Here's how the part is built. I have some questions about the finished solid (model axes, mm). A direction names the side the tool comes from. Give positions to 0.01 mm unless a question says otherwise; leave off trailing zeros. Loops run counter-clockwise (first coordinate to the right, second up) from the corner with the lowest first, then second, coordinate; pieces in that order, holes last. Notation, with made-up numbers: (-10, -4) - (9, -4) arc R25 cw to (9, 25) - close; hole circle Ø2 at (58.25, -26.5). An arc over 180 degrees is marked (long way). Use a Markdown table: item, result.
from build123d import *

# Parameters (mm, degrees)
SKETCH1_W                        = 113
SKETCH1_H                        = 107
MAIN_BODY_DEPTH                  = 5
SKETCH19_W                       = 18.5
SKETCH19_H                       = 18.5
BOSS_EXTRUDE1_DEPTH              = 3
SKETCH7_R                        = 3.5
SKETCH7_W                        = 80
SKETCH7_H                        = 51.5
SCREEN_AND_KNOB_LOCATATION_DEPTH = 79.220841213
SKETCH11_W                       = 67.654258951
SKETCH11_H                       = 30.527744354
INTERNAL_CAVITY_DEPTH            = 3
BOARDERS_OUTLINE_W               = 113
BOARDERS_OUTLINE_H               = 107
BOARDERS_DEPTH                   = 15
SKETCH6_R                        = 3.5
SCREW_HEAD_PLACEMENT_DEPTH       = 15
SKETCH10_R                       = 1.68009103
SKETCH10_R_2                     = 2
SCREW_HOLE_THROUGH_DEPTH         = 80.243296246
SKETCH14_W                       = 4.25
SKETCH14_H                       = 28
SD_CARD_SLOT_DEPTH               = 10
SKETCH15_R                       = 3
BUTTON_PRESS_DEPTH               = 8.25
GROOVE_CUT_DEPTH                 = 80.865511956
CANCEL_DECAL_DEPTH               = 1
MAIN_BODY_FILLET_R               = 4
SKETCH18_R                       = 7.625
CUT_EXTRUDE1_DEPTH               = 6.5


# Read off the part's stored shape, not the designer's step: Boarders
with BuildPart() as part:
    # Sketch1 → Main Body (new body)
    with BuildSketch(Plane.XY):
        Rectangle(SKETCH1_W, SKETCH1_H)
    extrude(amount=MAIN_BODY_DEPTH)

    # Sketch19 → Boss-Extrude1 (add)
    with BuildSketch(Plane(origin=(0, 0, 0), x_dir=(-1, 0, 0), z_dir=(0, 0, -1))):
        with Locations((-36.5, -34.5)):
            Rectangle(SKETCH19_W, SKETCH19_H)
    extrude(amount=BOSS_EXTRUDE1_DEPTH)

    # Sketch7 → Screen and knob locatation (cut, through all)
    with BuildSketch(Plane.XY.offset(5)):
        with Locations((36.3, -34.31)):
            Circle(SKETCH7_R)
        with Locations((-0.5, 9.25)):
            Rectangle(SKETCH7_W, SKETCH7_H)
    extrude(amount=-SCREEN_AND_KNOB_LOCATATION_DEPTH, mode=Mode.SUBTRACT)

    # Sketch11 → Internal cavity (cut)
    with BuildSketch(Plane(origin=(0, 0, 0), x_dir=(-1, 0, 0), z_dir=(0, 0, -1))):
        with Locations((6.575112586, -34.017474747)):
            Rectangle(SKETCH11_W, SKETCH11_H)
    extrude(amount=-INTERNAL_CAVITY_DEPTH, mode=Mode.SUBTRACT)

    # Boarders outline → Boarders (add)
    with BuildSketch(Plane(origin=(0, 0, 0), x_dir=(-1, 0, 0), z_dir=(0, 0, -1))):
        Rectangle(BOARDERS_OUTLINE_W, BOARDERS_OUTLINE_H)
        Polygon((-27.25201689, -49.281346924), (-27.25201689, -44.5), (-47.5, -44.5), (-47.5, 44.5), (47.5, 44.5), (47.5, -44.5), (40.402242061, -44.5), (40.402242061, -49.281346924), align=None, mode=Mode.SUBTRACT)
    extrude(amount=BOARDERS_DEPTH)

    # Sketch6 → Screw Head Placement (cut)
    with BuildSketch(Plane.XY.offset(5)):
        with Locations((-51.5, 48.5)):
            Circle(SKETCH6_R)
        with Locations((-51.5, -48.5)):
            Circle(SKETCH6_R)
        with Locations((51.5, -48.5)):
            Circle(SKETCH6_R)
        with Locations((51.5, 48.5)):
            Circle(SKETCH6_R)
    extrude(amount=-SCREW_HEAD_PLACEMENT_DEPTH, mode=Mode.SUBTRACT)

    # Sketch10 → Screw hole through (cut, through all)
    with BuildSketch(Plane.XY.offset(-10)):
        with Locations((-51.5, 48.5)):
            Circle(SKETCH10_R)
        with Locations((51.5, 48.5)):
            Circle(SKETCH10_R)
        with Locations((51.5, -48.5)):
            Circle(SKETCH10_R)
        with Locations((-51.5, -48.5)):
            Circle(SKETCH10_R_2)
    extrude(amount=-SCREW_HOLE_THROUGH_DEPTH, mode=Mode.SUBTRACT)

    # Sketch14 → SD Card Slot (cut)
    with BuildSketch(Plane.ZY.offset(56.5)):
        with Locations((-12.875, 8)):
            Rectangle(SKETCH14_W, SKETCH14_H)
    extrude(amount=-SD_CARD_SLOT_DEPTH, mode=Mode.SUBTRACT)

    # Sketch15 → Button Press (add)
    with BuildSketch(Plane(origin=(0, 0, 3), x_dir=(-1, 0, 0), z_dir=(0, 0, -1))):
        with Locations((-3.7199, -35.4101)):
            Circle(SKETCH15_R)
    extrude(amount=BUTTON_PRESS_DEPTH)

    # Sketch16 → Groove Cut (cut, through all)
    with BuildSketch(Plane(origin=(0, 0, 3), x_dir=(-1, 0, 0), z_dir=(0, 0, -1))):
        with BuildLine():
            Line((2.2801, -39.4101), (7.826420717, -39.4101))
            Line((7.826420717, -39.4101), (7.826420717, -39.9101))
            Line((7.826420717, -39.9101), (2.729589743, -39.9101))
            ThreePointArc((2.729589743, -39.9101), (1.86123883, -41.346591673), (0.2801, -41.9101))
            Line((0.2801, -41.9101), (-7.7199, -41.9101))
            ThreePointArc((-7.7199, -41.9101), (-9.487666953, -41.177866953), (-10.2199, -39.4101))
            Line((-10.2199, -39.4101), (-10.2199, -31.4101))
            ThreePointArc((-10.2199, -31.4101), (-9.487666953, -29.642333047), (-7.7199, -28.9101))
            Line((-7.7199, -28.9101), (0.2801, -28.9101))
            ThreePointArc((0.2801, -28.9101), (1.86123883, -29.473608327), (2.729589743, -30.9101))
            Line((2.729589743, -30.9101), (7.826420717, -30.9101))
            Line((7.826420717, -30.9101), (7.826420717, -31.4101))
            Line((7.826420717, -31.4101), (2.2801, -31.4101))
            ThreePointArc((2.2801, -31.4101), (1.694313562, -29.995886438), (0.2801, -29.4101))
            Line((0.2801, -29.4101), (-7.7199, -29.4101))
            ThreePointArc((-7.7199, -29.4101), (-9.134113562, -29.995886438), (-9.7199, -31.4101))
            Line((-9.7199, -31.4101), (-9.7199, -39.4101))
            ThreePointArc((-9.7199, -39.4101), (-9.134113562, -40.824313562), (-7.7199, -41.4101))
            Line((-7.7199, -41.4101), (0.2801, -41.4101))
            ThreePointArc((0.2801, -41.4101), (1.694313562, -40.824313562), (2.2801, -39.4101))
        make_face()
    extrude(amount=-GROOVE_CUT_DEPTH, mode=Mode.SUBTRACT)

    # Sketch17 → CAncel Decal (cut)
    with BuildSketch(Plane.XY.offset(5)):
        Polygon((0.356446609, -32.753753391), (3.012793219, -35.4101), (0.356446609, -38.066446609), (1.063553391, -38.773553391), (3.7199, -36.117206781), (6.376246609, -38.773553391), (7.083353391, -38.066446609), (4.427006781, -35.4101), (7.083353391, -32.753753391), (6.376246609, -32.046646609), (3.7199, -34.702993219), (1.063553391, -32.046646609), align=None)
    extrude(amount=-CANCEL_DECAL_DEPTH, mode=Mode.SUBTRACT)

    # Main Body Fillet
    main_body_fillet_edges = [part.edges().sort_by_distance(p)[0] for p in [
        (56.5, -53.5, -5),
        (-56.5, -53.5, -5),
        (-56.5, 53.5, -5),
        (56.5, 53.5, -5),
    ]]
    fillet(main_body_fillet_edges, radius=MAIN_BODY_FILLET_R)

    # Sketch18 → Cut-Extrude1 (cut)
    with BuildSketch(Plane.XY.offset(5)):
        with Locations((36.3, -34.31)):
            Circle(SKETCH18_R)
    extrude(amount=-CUT_EXTRUDE1_DEPTH, mode=Mode.SUBTRACT)


solid = part.part
(1) On a 3-axis mill with a long thin cutter (end or side, diameter ignored), from which of +Z, -Z, +X, -X, +Y, -Y can I reach the whole of each face in a straight line? I mean faces 1 (the face through (27.25, -35, -1)), 2 (the face through (-54.08, 50.865, -2.395)), 3 (the face through (-40.5, 9, 3)). Say none if no direction works.
A:
| item | result |
|---|---|
| face 1 | -Z |
| face 2 | +Z |
| face 3 | +Z, -Z |
(2) Suppose I cut it at D-D on x = 30. Write out the boundary of the cut face in (y, z), plus the area to 3 significant figures.
A:
| item | result |
|---|---|
| outline | (-53.5, -15) - (-44.5, -15) - (-44.5, 0) - (-43.75, 0) - (-43.75, -3) - (-25.25, -3) - (-25.25, 0) - (-16.5, 0) - (-16.5, 5) - (-30.01, 5) - (-30.01, -1.5) - (-38.61, -1.5) - (-38.61, 5) - (-53.5, 5) - close; (35, 0) - (44.5, 0) - (44.5, -15) - (53.5, -15) - (53.5, 5) - (35, 5) - close |
| area | 547 mm2 |
(3) Will these pins go through, and if not, where does the flat tip stop? pin 1 (3.5 mm diameter, centred on x = -51, y = 50, fed in from +Z); pin 2 (9 mm diameter, centred on x = 38.5, y = -30.5, fed in from -Z); pin 3 (7 mm diameter, centred on x = -52.5, y = 11.5, fed in from -Z); pin 4 (8 mm diameter, centred on x = 26.5, y = 29, fed in from +Z).
A:
| item | result |
|---|---|
| pin 1 | z = -10 |
| pin 2 | z = -3 |
| pin 3 | z = -10.75 |
| pin 4 | through |
(4) Suppose I cut it at A-A on y = -2.5. Write out the boundary of the cut face in (x, z), plus the area to 3 significant figures.
A:
| item | result |
|---|---|
| outline | (-56.5, -10.75) - (-47.5, -10.75) - (-47.5, 0) - (-40.5, 0) - (-40.5, 5) - (-56.5, 5) - close; (39.5, 0) - (47.5, 0) - (47.5, -15) - (56.5, -15) - (56.5, 5) - (39.5, 5) - close |
| area | 397 mm2 |
(5) We'd pull the mould along X, two halves only. Please class faces 4 (the face through (-55.297, 52.359, -4.86)), 5 (the face through (-52, -6, -13)), 6 (the face through (-6, -18.754, 1)): pulls with the +X half, pulls with the -X half, needs draft (parallel to the pull), parting line crosses it, or undercut.
A:
| item | result |
|---|---|
| face 4 | pulls with the -X half |
| face 5 | needs draft |
| face 6 | undercut |
(6) Suppose I cut it at B-B on x = -15.5. Write out the boundary of the cut face in (y, z).
A:
| item | result |
|---|---|
| outline | (-53.5, -15) - (-49.28, -15) - (-49.28, 3) - (-18.75, 3) - (-18.75, 0) - (-16.5, 0) - (-16.5, 5) - (-53.5, 5) - close; (35, 0) - (44.5, 0) - (44.5, -15) - (53.5, -15) - (53.5, 5) - (35, 5) - close |
(7) If I drill on line 1 (Y direction, x = -51.5, z = -4.25); line 2 (Y direction, x = -39, z = 2); line 3 (Y direction, x = -39, z = -10.25), over which ranges is the centre line in solid material (lowest first)?
A:
| item | result |
|---|---|
| line 1 | -53.5 to -52, -45 to 45, 52 to 53.5 |
| line 2 | -53.5 to -49.28, -18.75 to -16.5, 35 to 53.5 |
| line 3 | -53.5 to -49.28, 44.5 to 53.5 |
(8) Suppose I cut it at C-C on z = -12.5. Write out the boundary of the cut face in (x, y).
A:
| item | result |
|---|---|
| outline | (-56.5, -49.5) arc R4 ccw to (-52.5, -53.5) - (52.5, -53.5) arc R4 ccw to (56.5, -49.5) - (56.5, 49.5) arc R4 ccw to (52.5, 53.5) - (-52.5, 53.5) arc R4 ccw to (-56.5, 49.5) - (-56.5, 22) - (-47.5, 22) - (-47.5, 44.5) - (47.5, 44.5) - (47.5, -44.5) - (27.25, -44.5) - (27.25, -49.28) - (-40.4, -49.28) - (-40.4, -44.5) - (-47.5, -44.5) - (-47.5, -6) - (-56.5, -6) - close; hole circle Ø4 at (-51.5, -48.5); hole circle Ø3.36 at (-51.5, 48.5); hole circle Ø3.36 at (51.5, -48.5); hole circle Ø3.36 at (51.5, 48.5) |
